```python
from build123d import *

# Parameters (mm, degrees)
SKETCH1_W           = 70
SKETCH1_H           = 50
BOSS_EXTRUDE1_DEPTH = 50
CUT_EXTRUDE1_DEPTH  = 50
CUT_EXTRUDE2_DEPTH  = 50
CUT_EXTRUDE3_DEPTH  = 10
CUT_EXTRUDE4_DEPTH  = 57


with BuildPart() as part:
    # Sketch1 → Boss-Extrude1 (new body)
    with BuildSketch(Plane.XY):
        with Locations((35, 25)):
            Rectangle(SKETCH1_W, SKETCH1_H)
    extrude(amount=BOSS_EXTRUDE1_DEPTH)

    # Sketch2 → Cut-Extrude1 (cut)
    with BuildSketch(Plane.XY.offset(50)):
        Polygon((0, 10), (10, 10), (20, 20), (20, 50), (0, 50), align=None)
    extrude(amount=-CUT_EXTRUDE1_DEPTH, mode=Mode.SUBTRACT)

    # Sketch3 → Cut-Extrude2 (cut)
    with BuildSketch(Plane.XZ):
        Polygon((0, 20), (60, 50), (0, 50), align=None)
    extrude(amount=-CUT_EXTRUDE2_DEPTH, mode=Mode.SUBTRACT)

    # Sketch4 → Cut-Extrude3 (cut)
    with BuildSketch(Plane(origin=(0, 50, 0), x_dir=(1, 0, 0), z_dir=(0, 1, 0))):
        Polygon((20, -10), (50, -10), (50, -30), (70, -30), (70, -50), (60, -50), (20, -30), align=None)
    extrude(amount=-CUT_EXTRUDE3_DEPTH, mode=Mode.SUBTRACT)

    # Sketch5 → Cut-Extrude4 (cut)
    with BuildSketch(Plane.XY.offset(10)):
        Polygon((20, 20), (40, 40), (20, 40), align=None)
    extrude(amount=CUT_EXTRUDE4_DEPTH, mode=Mode.SUBTRACT)


solid = part.part
```
The listing builds one solid part. Answer for the finished solid, in the listing's coordinates (mm). A direction names the side the tool comes from. Round coordinates to 2 decimals unless told otherwise and drop trailing zeros. Loops run counter-clockwise (first coordinate to the right, second up) from the corner with the lowest first, then second, coordinate; pieces in that order, holes last. Notation, with made-up numbers: (79, 55.25) - (112, 55.25) arc R32 cw to (112, 88.25) - close; hole circle Ø4 at (51, 6.25). An arc over 180 degrees is marked (long way). Use one line per item in the form item = value. Start each with the question number.
1. For a pull along X with two mould halves and no side action, classify faces 6 (the face through (5, 10, 13)), 7 (the face through (50, 45, 20)), 8 (the face through (70, 25, 25)) as pulls with the +X half, pulls with the -X half, needs draft (parallel to the pull), parting line crosses it, or undercut.
2. The part is cut by section A-A on y = 33. Determine the outline of the cut face in (x, z), then the cut area to 3 significant figures.
3. Given pin 1 Ø5 at (y, z) = (44.5, 17) entering from -X; pin 2 Ø1.5 at (x, z) = (29.5, 5.5) entering from -Y; pin 3 Ø6 at (y, z) = (18, 15) entering from -X; pin 4 Ø11 at (x, z) = (5, 15) entering from +Y, each flat-ended and moving along its own axis, determine where each tip first touches the part or whether it passes through.
4. The part is cut by section B-B on z = 4. Determine the outline of the cut face in (x, y), then the cut area to 3 significant figures.
5. The part is cut by section D-D on z = 18. Determine the outline of the cut face in (x, y).
6. Consider line 1 (Y direction, x = 6.5, z = 8); line 2 (X direction, y = 9, z = 30). Determine where each line is inside the solid, lowest interval first. Write a range as [from, to].
7. A tool of negligible diameter and unlimited length cuts with its end or side. For faces 1 (the face through (0, 5, 10)), 2 (the face through (31, 39, 10)), 3 (the face through (60, 45, 30)), 4 (the face through (20, 35, 5)), 5 (the face through (42, 25, 0)), from which of +Z, -Z, +X, -X, +Y, -Y can it reach the whole face along a straight path? Write none if from no direction.
8. The part is cut by section C-C on x = 27. Determine the outline of the cut face in (y, z).
Geometry check:
q1.face_6 = needs draft
q1.face_7 = pulls with the -X half
q1.face_8 = pulls with the +X half
q2.outline = (20, 0) - (70, 0) - (70, 50) - (60, 50) - (33, 36.5) - (33, 10) - (20, 10) - close
q2.area = 1,800 mm^2
q3.pin_1 = 50
q3.pin_2 = 0
q3.pin_3 = 15
q3.pin_4 = 10.5
q4.outline = (0, 0) - (70, 0) - (70, 50) - (20, 50) - (20, 20) - (10, 10) - (0, 10) - close
q4.area = 2,750 mm^2
q5.outline = (0, 0) - (70, 0) - (70, 50) - (50, 50) - (50, 40) - (40, 40) - (10, 10) - (0, 10) - close
q6.line_1 = [0, 10]
q6.line_2 = [20, 70]
q7.face_1 = +Z, -Z, -X, +Y, -Y
q7.face_2 = +Z, -X, +Y
q7.face_3 = +Z, +X, -X, +Y
q7.face_4 = +Z, -Z, -X, +Y
q7.face_5 = -Z, +X, -X, +Y, -Y
q8.outline = (0, 0) - (50, 0) - (50, 10) - (27, 10) - (27, 33.5) - (0, 33.5) - close
